Can you work these out from the model? Positions are in its coordinate system, mm. A direction names the side the tool comes from. Give positions to 0.01 mm unless a question says otherwise; leave off trailing zeros. Loops run counter-clockwise (first coordinate to the right, second up) from the corner with the lowest first, then second, coordinate; pieces in that order, holes last. Notation, with made-up numbers: M 74.5,86 L 108.5,86 A19 cw 108.5,95 Z; hole C 66,23.25 d10. An arc over 180 degrees is marked long. Answer as a JSON object with one key per item and string values.
```python
from build123d import *
from build123d.topology import SkipClean

# Parameters (mm, degrees)
SKETCH1_R                            = 94
SKETCH1_R_2                          = 90
BOSS_EXTRUDE1_DEPTH                  = 50
BOSS_EXTRUDE2_REACH                  = 144.028
BOSS_EXTRUDE2_END_RADIUS             = 90
SKETCH2_W                            = 70
SKETCH2_H                            = 70
BOSS_EXTRUDE2_DIRECTION_2_REACH      = 144.028
BOSS_EXTRUDE2_DIRECTION_2_END_RADIUS = 90
CUT_EXTRUDE1_DEPTH                   = 143.028166221
CUT_EXTRUDE1_DEPTH_BACK              = 143.028166221
CUT_EXTRUDE3_DEPTH                   = 143.028166221
CUT_EXTRUDE3_DEPTH_BACK              = 143.028166221
SKETCH2_3_R                          = 1


with BuildPart() as part:
    # Sketch1 → Boss-Extrude1 (new, symmetric)
    with BuildSketch(Plane(origin=(0, 0, 0), x_dir=(1, 0, 0), z_dir=(0, 1, 0))):
        with Locations(Location((0, 0, 0), (0, 0, 270))):
            Circle(SKETCH1_R)
        with Locations(Location((0, 0, 0), (0, 0, 270))):
            Circle(SKETCH1_R_2, mode=Mode.SUBTRACT)
    extrude(amount=BOSS_EXTRUDE1_DEPTH, both=True)

    # Boss-Extrude2: up to this cylinder (the profile starts inside it)
    boss_extrude2_end = Plane(origin=(0, 0, 0), z_dir=(0, -1, 0)) * Cylinder(BOSS_EXTRUDE2_END_RADIUS, 469.056, mode=Mode.PRIVATE)
    # Sketch2 → Boss-Extrude2 (add, up to the surface)
    with BuildSketch(Plane(origin=(0, 0, 0), x_dir=(0, 0, -1), z_dir=(1, 0, 0)), mode=Mode.PRIVATE) as boss_extrude2_sk1:
        Rectangle(SKETCH2_W, SKETCH2_H)
    boss_extrude2_tool1 = extrude(boss_extrude2_sk1.sketch, amount=-BOSS_EXTRUDE2_REACH, mode=Mode.PRIVATE) & boss_extrude2_end
    add(boss_extrude2_tool1.solids().sort_by_distance((0, 0, 0))[0])

    # Boss-Extrude2 direction 2: up to this cylinder (the profile starts inside it)
    boss_extrude2_direction_2_end = Plane(origin=(0, 0, 0), z_dir=(0, -1, 0)) * Cylinder(BOSS_EXTRUDE2_DIRECTION_2_END_RADIUS, 469.056, mode=Mode.PRIVATE)
    # Sketch2 → Boss-Extrude2 direction 2 (add, up to the surface)
    with BuildSketch(Plane(origin=(0, 0, 0), x_dir=(0, 0, -1), z_dir=(1, 0, 0)), mode=Mode.PRIVATE) as boss_extrude2_direction_2_sk1:
        Rectangle(SKETCH2_W, SKETCH2_H)
    boss_extrude2_direction_2_tool1 = extrude(boss_extrude2_direction_2_sk1.sketch, amount=BOSS_EXTRUDE2_DIRECTION_2_REACH, mode=Mode.PRIVATE) & boss_extrude2_direction_2_end
    add(boss_extrude2_direction_2_tool1.solids().sort_by_distance((0, 0, 0))[0])

    # Sketch3 → Cut-Extrude1 (cut, two sides: drawn at the far end of the back side and taken through both)
    with SkipClean():  # the faces are left unmerged after this step: merging them gives an invalid solid
        with BuildSketch(Plane(origin=(0, 0, 0), x_dir=(1, 0, 0), z_dir=(0, 1, 0)).offset(-CUT_EXTRUDE1_DEPTH_BACK)):
            with BuildLine():
                Line((-85, 29.580398915), (-85, -29.580398915))
                ThreePointArc((-85, -29.580398915), (0, -90), (85, -29.580398915))
                Line((85, -29.580398915), (85, 29.580398915))
                ThreePointArc((85, 29.580398915), (0, 90), (-85, 29.580398915))
            make_face()
        extrude(amount=CUT_EXTRUDE1_DEPTH + CUT_EXTRUDE1_DEPTH_BACK, mode=Mode.SUBTRACT)

    # Sketch2_3 → Cut-Extrude3 (cut, two sides: drawn at the far end of the back side and taken through both)
    with SkipClean():  # the faces are left unmerged after this step: merging them gives an invalid solid
        with BuildSketch(Plane(origin=(0, 0, 0), x_dir=(0, 0, -1), z_dir=(1, 0, 0)).offset(-CUT_EXTRUDE3_DEPTH_BACK)):
            with Locations((10.606601718, 10.606601718)):
                Circle(SKETCH2_3_R)
            with Locations((-10.606601718, 10.606601718)):
                Circle(SKETCH2_3_R)
            with Locations((-10.606601718, -10.606601718)):
                Circle(SKETCH2_3_R)
            with Locations((10.606601718, -10.606601718)):
                Circle(SKETCH2_3_R)
        extrude(amount=CUT_EXTRUDE3_DEPTH + CUT_EXTRUDE3_DEPTH_BACK, mode=Mode.SUBTRACT)


solid = part.part
```
1) Suppose I cut it at D-D, the plane z = 52. Write out the boundary of the cut face in (x, y), and give its area (3 significant figures).
Answer list:
{"outline": "M -78.31,-50 L -73.46,-50 L -73.46,50 L -78.31,50 Z; M 73.46,-50 L 78.31,-50 L 78.31,50 L 73.46,50 Z", "area": "970 mm^2"}
2) For faces 4 (the flat face through (-87, -35, 0)), 5 (the flat face through (-85, 0, 0)), 6 (the flat face through (-87, 35, 0)), which set-ups out of +Z, -Z, +X, -X, +Y, -Y let a thin tool reach every point of the face, with its end or its side?
Answer list:
{"face 4": "-Y", "face 5": "+Y, -Y", "face 6": "+Y"}
3) Suppose I cut it at C-C, the plane x = -63. Write out the boundary of the cut face in (y, z), and give its area (3 significant figures).
Answer list:
{"outline": "M -50,-69.76 L 50,-69.76 L 50,-64.27 L -50,-64.27 Z; M -50,64.27 L 50,64.27 L 50,69.76 L -50,69.76 Z", "area": "1,100 mm^2"}
4) Will these pins go through, and if not, where does the flat tip stop? pin 1 Ø2 at (y, z) = (14.5, 24) entering from +X; pin 2 Ø2.5 at (y, z) = (-10.61, 10.61) entering from -X; pin 3 Ø2.5 at (x, z) = (-87, 10.5) entering from +Y; pin 4 Ø5.5 at (x, z) = (-86.5, -12) entering from -Y.
Answer list:
{"pin 1": "x = 91.14", "pin 2": "x = -93.53", "pin 3": "y = 35", "pin 4": "y = -50"}
5) If we mould it in two halves opening along Z, with no side actions, what happens to faces 1 (the flat face through (87, -35, 0)), 2 (the cylindrical face through (63.53, 0.7, -69.28)), 3 (the flat face through (-48.3, 50, 76.2))? For each: +Z half, -Z half, draft (parallel to the pull), parting line (faces both ways), or undercut.
Answer list:
{"face 1": "undercut", "face 2": "parting line", "face 3": "draft"}
6) Please list where these lines run through material, in increasing order: line 1 along Z through (x, y) = (-9.5, 45); line 2 along Z through (x, y) = (-77, -42); line 3 along X through (y, z) = (-44.5, -37). Write a range as from..to.
Answer list:
{"line 1": "-93.52..-89.5, 89.5..93.52", "line 2": "-53.92..-46.59, 46.59..53.92", "line 3": "-86.41..-82.04, 82.04..86.41"}
7) Suppose I cut it at B-B, the plane y = 0.5. Write out the boundary of the cut face in (x, z).
Answer list:
{"outline": "C 0,0 d188; hole M -85,-29.58 A90 ccw 85,-29.58 L 85,29.58 A90 ccw -85,29.58 Z"}
8) Suppose I cut it at A-A, the plane z = 0. Write out the boundary of the cut face in (x, y), and give its area (3 significant figures).
Answer list:
{"outline": "M -94,-50 L -90,-50 L -90,-35 L -85,-35 L -85,35 L -90,35 L -90,50 L -94,50 Z; M 85,-35 L 90,-35 L 90,-50 L 94,-50 L 94,50 L 90,50 L 90,35 L 85,35 Z", "area": "1,500 mm^2"}
